Geometry check sheet. Reference: the model listing, model coordinates, mm. Face numbers are marked on the shaded views. A direction names the side the tool comes from. Round coordinates to 2 decimals unless told otherwise and drop trailing zeros. Order: outer loops, then holes, each group sorted by start corner. A loop starts at its lowest first (then second) coordinate and runs counter-clockwise, first axis right, second up. Notation, with made-up numbers: (62, 0) - (84, 0) arc R20 cw to (84, 25) - close; hole circle Ø9 at (-36, -10.75). An arc over 180 degrees is marked (long way). Return JSON: item names as keys, results as strings. Group by question number.
Q1. Tool access check on the marked faces 1, 2, 3 and 4. Record the directions out of +Z, -Z, +X, -X, +Y, -Y that give a thin tool (end or side, any length) a straight path to the whole face; none if there is none.
Q2. Sectioned sample at D-D, the plane x = -15. Record the cut outline in (y, z), then the cut area to 3 significant figures.
Q3. Sectioned sample at C-C, the plane y = -28. Record the cut outline in (x, z).
Q4. Gauge pin test, flat ends, axial feed: pin 1 Ø4.5 at (x, y) = (-21.5, -27) entering from +Z; pin 2 Ø1.5 at (x, z) = (-15, 1.5) entering from -Y; pin 3 Ø5.5 at (y, z) = (-3, 11) entering from +X. Record the tip position at first contact, or that the pin passes through.
Q5. Material ranges on line 1 along X through (y, z) = (-9.5, 4); line 2 along Y through (x, z) = (9, 9.5); line 3 along Z through (x, y) = (-16, -2.75), recorded low to high.
Q6. Draft check along X on the marked faces 5, 6, 7 and 8. Enter one of: pulls with the +X half, pulls with the -X half, needs draft (parallel to the pull), parting line crosses it, or undercut.
Q7. Sectioned sample at A-A, the plane z = 6. Record the cut outline in (x, y).
Q8. Sectioned sample at B-B, the plane x = 16. Record the cut outline in (y, z).
```python
from build123d import *

# Parameters (mm, degrees)
SKETCH_R        = 1.8
PAD_DEPTH       = 7
SKETCH001_R     = 2.9
POCKET_DEPTH    = 3
SKETCH002_W     = 11.4
SKETCH002_H     = 5
PAD001_DEPTH    = 6
SKETCH005_R     = 1.8
POCKET002_DEPTH = 5
SKETCH003_W     = 20.2
SKETCH003_H     = 13
PAD002_DEPTH    = 6
SKETCH009_W     = 12.2
SKETCH009_H     = 13
POCKET006_DEPTH = 9.6
POCKET003_DEPTH = 47.001
POCKET004_DEPTH = 5
POCKET005_DEPTH = 3.2


with BuildPart() as part:
    # Sketch → Pad (new body)
    with BuildSketch(Plane.XY):
        with BuildLine():
            Line((-21.5, 0), (-21.5, -5))
            Line((-21.5, -5), (-10.1, -5))
            Line((-10.1, -5), (-10.1, -18))
            ThreePointArc((-12.291233, -20.888926), (-10.70978, -19.812967), (-10.1, -18))
            Line((-12.291233, -20.888926), (-22.213151, -23.666611))
            ThreePointArc((-22.213151, -23.666611), (-24.933961, -30.184937), (-17.962388, -31.320077))
            Line((-7.112537, -21.393308), (-17.962388, -31.320077))
            ThreePointArc((-6.1, -21), (-6.643121, -21.10178), (-7.112537, -21.393308))
            Line((-6.1, -21), (6.1, -21))
            ThreePointArc((7.112537, -21.393308), (6.643121, -21.10178), (6.1, -21))
            Line((7.112537, -21.393308), (17.962388, -31.320077))
            ThreePointArc((17.962388, -31.320077), (24.933961, -30.184937), (22.213151, -23.666611))
            Line((12.291233, -20.888926), (22.213151, -23.666611))
            ThreePointArc((10.1, -18), (10.70978, -19.812967), (12.291233, -20.888926))
            Line((10.1, -5), (10.1, -18))
            Line((21.5, -5), (10.1, -5))
            Line((21.5, -5), (21.5, 0))
            Line((21.5, 0), (6.1, 0))
            Line((6.1, 0), (6.1, -8))
            Line((-6.1, -8), (6.1, -8))
            Line((-6.1, 0), (-6.1, -8))
            Line((-21.5, 0), (-6.1, 0))
        make_face()
        with Locations((-21, -28)):
            Circle(SKETCH_R, mode=Mode.SUBTRACT)
        with Locations((21, -28)):
            Circle(SKETCH_R, mode=Mode.SUBTRACT)
    extrude(amount=PAD_DEPTH)

    # Sketch001 (on Face26 of Pad) → Pocket (cut)
    with BuildSketch(Plane.XY.offset(7)):
        with Locations((-21, -28)):
            Circle(SKETCH001_R)
        with Locations((21, -28)):
            Circle(SKETCH001_R)
    extrude(amount=-POCKET_DEPTH, mode=Mode.SUBTRACT)

    # Sketch002 (on Face5 of Pocket) → Pad001 (join)
    with BuildSketch(Plane.XY.offset(7)):
        with Locations((15.8, -2.5)):
            Rectangle(SKETCH002_W, SKETCH002_H)
        with Locations((-15.8, -2.5)):
            Rectangle(SKETCH002_W, SKETCH002_H)
    extrude(amount=PAD001_DEPTH)

    # Sketch005 (on Face30 of Pad001) → Pocket002 (cut)
    with BuildSketch(Plane(origin=(0, 0, 0), x_dir=(-1, 0, 0), z_dir=(0, 1, 0))):
        with Locations((-16, 9)):
            Circle(SKETCH005_R)
        with Locations((16, 9)):
            Circle(SKETCH005_R)
    extrude(amount=-POCKET002_DEPTH, mode=Mode.SUBTRACT)

    # Sketch003 (on Face3 of Pad001) → Pad002 (join)
    with BuildSketch(Plane.XY.offset(7)):
        with Locations((0, -14.5)):
            Rectangle(SKETCH003_W, SKETCH003_H)
    extrude(amount=PAD002_DEPTH)

    # Sketch009 (on Face1 of Pad002) → Pocket006 (cut)
    with BuildSketch(Plane(origin=(0, 0, 0), x_dir=(1, 0, 0), z_dir=(0, 0, -1))):
        with Locations((0, 14.5)):
            Rectangle(SKETCH009_W, SKETCH009_H)
    extrude(amount=-POCKET006_DEPTH, mode=Mode.SUBTRACT)

    # Sketch006 → Pocket003 (cut, through all)
    with BuildSketch(Plane(origin=(-21.5, 0, 0), x_dir=(0, -1, 0), z_dir=(-1, 0, 0))):
        Polygon((5, 0), (0, 0), (0, 5), align=None)
    extrude(amount=-POCKET003_DEPTH, mode=Mode.SUBTRACT)

    # Sketch007 (on Face29 of Pocket003) → Pocket004 (cut)
    with BuildSketch(Plane.XZ.offset(5)):
        Polygon((-21.5, 0), (-21.5, 9), (-12.5, 0), align=None)
        Polygon((21.5, 0), (21.5, 9), (12.5, 0), align=None)
    extrude(amount=-POCKET004_DEPTH, mode=Mode.SUBTRACT)

    # Sketch008 (on Face18 of Pocket004) → Pocket005 (cut)
    with BuildSketch(Plane.XY.offset(13)):
        with BuildLine():
            ThreePointArc((1.8, -12), (0, -10.2), (-1.8, -12))
            Line((-1.8, -12), (-1.8, -16))
            ThreePointArc((-1.8, -16), (0, -17.8), (1.8, -16))
            Line((1.8, -12), (1.8, -16))
        make_face()
    extrude(amount=-POCKET005_DEPTH, mode=Mode.SUBTRACT)


solid = part.part
```
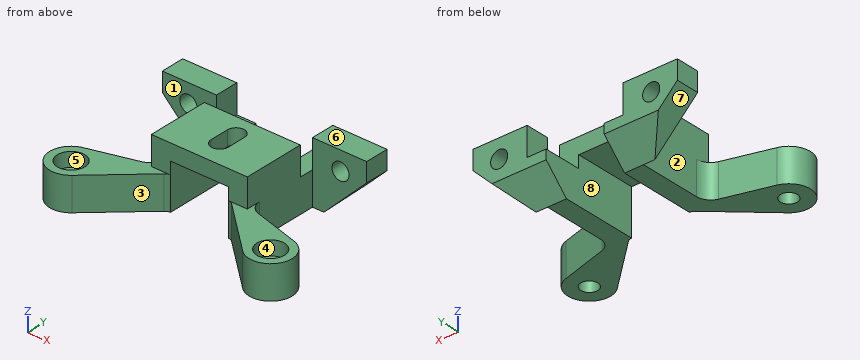
Reply:
{
 "1": {"face 1": "+Z, -Z, -X", "face 2": "+Z, -X", "face 3": "+Z, -Z, -Y", "face 4": "+Z"},
 "2": {"outline": "(-28.61, 0) - (-21.65, 0) - (-21.65, 7) - (-28.61, 7) - close; (-5, 2.5) - (-2.5, 2.5) - (0, 5) - (0, 7.5) - (-5, 7.5) - close; (-5, 10.5) - (0, 10.5) - (0, 13) - (-5, 13) - close", "area": "83.1 mm^2"},
 "3": {"outline": "(-25.5, 0) - (-22.8, 0) - (-22.8, 4) - (-23.9, 4) - (-23.9, 7) - (-25.5, 7) - close; (-19.2, 0) - (-14.33, 0) - (-14.33, 7) - (-18.1, 7) - (-18.1, 4) - (-19.2, 4) - close; (14.33, 0) - (19.2, 0) - (19.2, 4) - (18.1, 4) - (18.1, 7) - (14.33, 7) - close; (22.8, 0) - (25.5, 0) - (25.5, 7) - (23.9, 7) - (23.9, 4) - (22.8, 4) - close"},
 "4": {"pin 1": "z = 7", "pin 2": "y = -29.3", "pin 3": "x = 21.5"},
 "5": {"line 1": "-10.1 to -6.1, 6.1 to 10.1", "line 2": "-21 to -8", "line 3": "3.5 to 7.2, 10.8 to 13"},
 "6": {"face 5": "undercut", "face 6": "needs draft", "face 7": "pulls with the -X half", "face 8": "undercut"},
 "7": {"outline": "(-22.21, -23.67) arc R4.5 ccw (long way) to (-17.96, -31.32) - (-7.11, -21.39) arc R1.5 cw to (-6.1, -21) - (-6.1, 0) - (-18.5, 0) - (-18.5, -5) - (-10.1, -5) - (-10.1, -18) arc R3 cw to (-12.29, -20.89) - close; (6.1, -21) arc R1.5 cw to (7.11, -21.39) - (17.96, -31.32) arc R4.5 ccw (long way) to (22.21, -23.67) - (12.29, -20.89) arc R3 cw to (10.1, -18) - (10.1, -5) - (18.5, -5) - (18.5, 0) - (6.1, 0) - close; hole circle Ø5.8 at (-21, -28); hole circle Ø5.8 at (21, -28)"},
 "8": {"outline": "(-29.52, 0) - (-21.93, 0) - (-21.93, 7) - (-29.52, 7) - close; (-5, 3.5) - (-1.5, 3.5) - (0, 5) - (0, 7.2) - (-5, 7.2) - close; (-5, 10.8) - (0, 10.8) - (0, 13) - (-5, 13) - close"}
}
